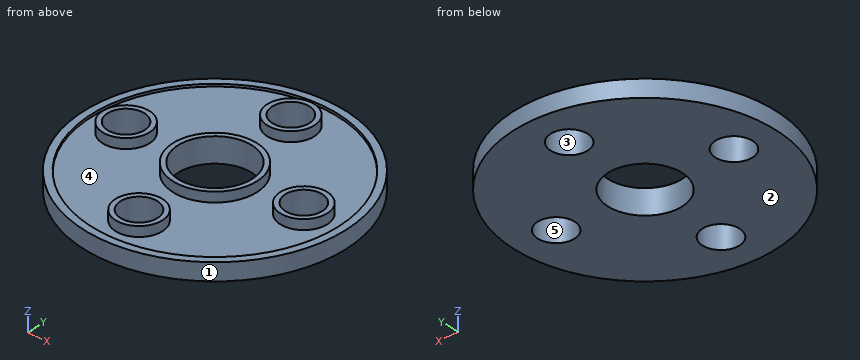
```python
from build123d import *

# Parameters (mm, degrees)
F0_R     = 53
F0_R_2   = 50
F1_DEPTH = 7
F0_R_3   = 9.5
F0_R_4   = 17
F2_DEPTH = 6
F0_R_5   = 7.5
F0_R_6   = 15
F3_DEPTH = 10


with BuildPart() as f1:
    # F0 (on Top) → F1 (new body)
    with BuildSketch(Plane.XY):
        Circle(F0_R)
        Circle(F0_R_2, mode=Mode.SUBTRACT)
    extrude(amount=F1_DEPTH)

    # F0 (on Top) → F2 (join)
    with BuildSketch(Plane.XY):
        Circle(F0_R)
        Circle(F0_R_2, mode=Mode.SUBTRACT)
        Circle(F0_R_2)
        with Locations((0, -36)):
            Circle(F0_R_3, mode=Mode.SUBTRACT)
        with Locations((-36, 0)):
            Circle(F0_R_3, mode=Mode.SUBTRACT)
        Circle(F0_R_4, mode=Mode.SUBTRACT)
        with Locations((36, 0)):
            Circle(F0_R_3, mode=Mode.SUBTRACT)
        with Locations((0, 36)):
            Circle(F0_R_3, mode=Mode.SUBTRACT)
    extrude(amount=F2_DEPTH)

    # F0 (on Top) → F3 (join)
    with BuildSketch(Plane.XY):
        with Locations((0, 36)):
            Circle(F0_R_3)
        with Locations((0, 36)):
            Circle(F0_R_5, mode=Mode.SUBTRACT)
        with Locations((36, 0)):
            Circle(F0_R_3)
        with Locations((36, 0)):
            Circle(F0_R_5, mode=Mode.SUBTRACT)
        with Locations((-36, 0)):
            Circle(F0_R_3)
        with Locations((-36, 0)):
            Circle(F0_R_5, mode=Mode.SUBTRACT)
        with Locations((0, -36)):
            Circle(F0_R_3)
        with Locations((0, -36)):
            Circle(F0_R_5, mode=Mode.SUBTRACT)
        Circle(F0_R_4)
        Circle(F0_R_6, mode=Mode.SUBTRACT)
    extrude(amount=F3_DEPTH)


solid = f1.part
```
Check sheet for the modelled part. Datum: model origin and axes. Units: mm. Face numbers are marked on the shaded views. A direction names the side the tool comes from. Coordinates: 2 decimals unless noted, no trailing zeros. Order: outer loops, then holes, each group sorted by start corner. A loop starts at its lowest first (then second) coordinate and runs counter-clockwise, first axis right, second up. Notation, with made-up numbers: M 89,75.25 L 103,75.25 A12 ccw 103,82.25 Z; hole C -8,0 d2. An arc over 180 degrees is marked long. Write each question's results on one line, items separated by ' | '. Start each with the question number.
1. Mould release check, pull along X, two halves, no side actions. Record for the marked faces 1, 2 and 3: +X half, -X half, draft (parallel to the pull), parting line (faces both ways), or undercut.
2. Go/stop test with flat-tipped pins: P1, Ø13.5, axis at x = -36, y = 0, coming from the +Z side; P2, Ø1, axis at y = 13.5, z = 3, coming from the -X side; P3, Ø2, axis at y = -30, z = 4.5, coming from the -X side; P4, Ø4, axis at x = 13, z = 1, coming from the -Y side. Record where each tip stops, or that it passes through.
3. Cross-section at B-B on x = -34.5. Record the cut outline in (y, z).
4. Cross-section at D-D on y = -36. Record the cut outline in (x, z), and give its area (3 significant figures).
5. Access from +Z, -Z, +X, -X, +Y, -Y to the whole of each face (thin tool, end or side, straight path). Record for the marked faces 4 and 5.
6. Cross-section at C-C on z = 4.75. Record the cut outline in (x, y), and give its area (3 significant figures).
7. Material ranges on probe 1 along Z at (x, y) = (-18, 26); probe 2 along X at (y, z) = (6.5, 1.75); probe 3 along X at (y, z) = (2, 8), recorded low to high.
8. Cross-section at A-A on y = 0. State how many separate pieces and enclosed holes the cut face has, and give its area (3 significant figures).
Checks:
1) face 1: parting line | face 2: draft | face 3: undercut
2) P1: passes through | P2: stops at x = -51.38 | P3: stops at x = -44.36 | P4: stops at y = -51.85
3) outline: M -40.23,0 L -7.35,0 L -7.35,10 L -9.38,10 L -9.38,6 L -36.19,6 L -36.19,7 L -40.23,7 Z; M 7.35,0 L 40.23,0 L 40.23,7 L 36.19,7 L 36.19,6 L 9.38,6 L 9.38,10 L 7.35,10 Z
4) outline: M -38.9,0 L -7.5,0 L -7.5,10 L -9.5,10 L -9.5,6 L -34.7,6 L -34.7,7 L -38.9,7 Z; M 7.5,0 L 38.9,0 L 38.9,7 L 34.7,7 L 34.7,6 L 9.5,6 L 9.5,10 L 7.5,10 Z | area: 401 mm²
5) face 4: +Z | face 5: +Z, -Z
6) outline: C 0,0 d106; hole C -36,0 d15; hole C 0,0 d30; hole C 0,-36 d15; hole C 0,36 d15; hole C 36,0 d15 | area: 7,410 mm²
7) probe 1: z = 0 to 6 | probe 2: x = -52.6 to -39.74, -32.26 to -13.52, 13.52 to 32.26, 39.74 to 52.6 | probe 3: x = -45.29 to -43.23, -28.77 to -26.71, -16.88 to -14.87, 14.87 to 16.88, 26.71 to 28.77, 43.23 to 45.29
8) separate pieces: 4 | enclosed holes: 0 | area: 330 mm²
